Drawing for the job (mm, zero at the part's lowest x, y, z). A direction names the side the tool comes from. Round coordinates to 2 decimals unless told otherwise and drop trailing zeros. Write each loop counter-clockwise with the first axis right and the second up, starting at its lowest first coordinate (ties: lowest second). Pieces come first, ordered by that corner, then holes. Notation, with made-up numbers: (44, 66) - (52, 66) arc R31 cw to (52, 102) - close; hole circle Ø11 at (31.25, 47.5). An arc over 180 degrees is marked (long way). One line per question, with ' | ' between items.
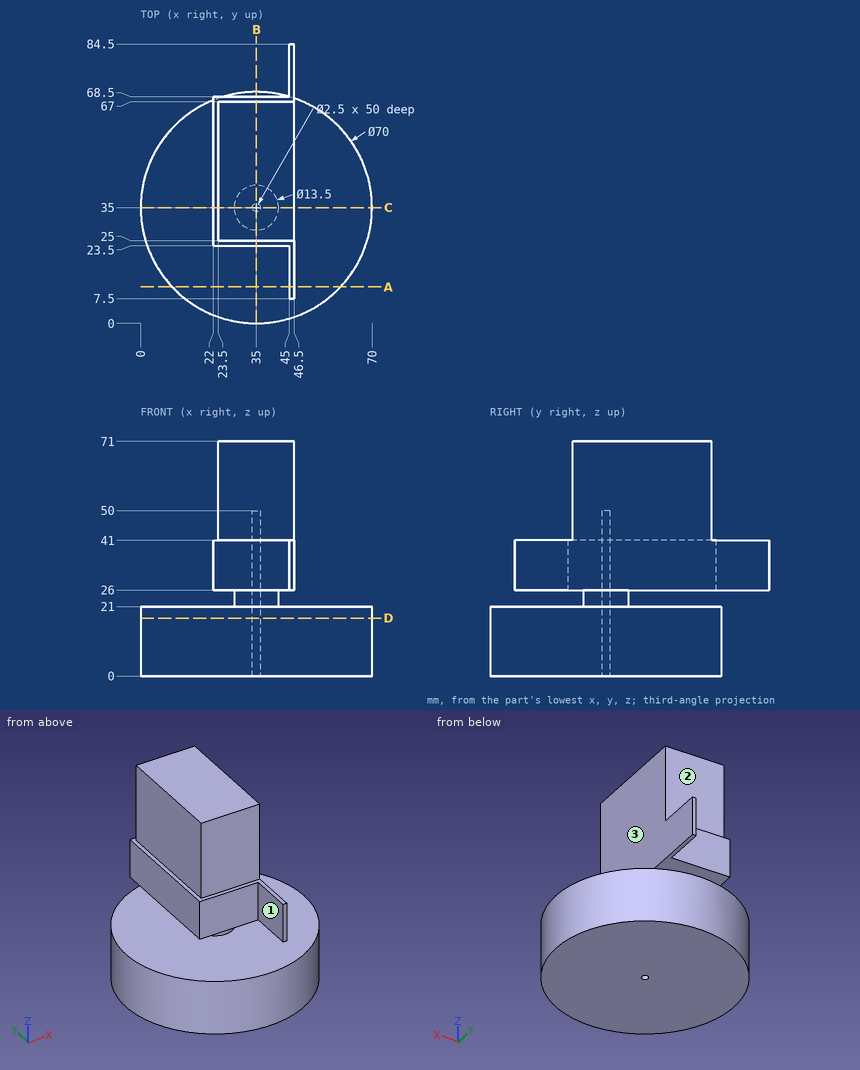
Q1. Drill centre lines: L1, parallel to Z at x = 43.5, y = 35.5; L2, parallel to Y at x = 35, z = 19; L3, parallel to Y at x = 35, z = 38. Where is each one in solid material? Low to high. Write a range as from..to.
Found:
L1: 0..21, 26..71 | L2: 0..33.75, 36.25..70 | L3: 23.5..33.75, 36.25..68.5
Q2. Which spindle directions (+Z, -Z, +X, -X, +Y, -Y) get a long thin tool onto all of the face, cutting with end or side? Do the marked faces 1, 2 and 3. Say none if no direction does.
Found:
face 1: +Z, -X, -Y | face 2: +Z, +X, -X, +Y | face 3: +Z, +X, +Y, -Y
Q3. Saw through at C-C, the plane y = 35. List the corners of the cut face in (x, z).
Found:
outline: (0, 0) - (33.75, 0) - (33.75, 50) - (36.25, 50) - (36.25, 0) - (70, 0) - (70, 21) - (41.75, 21) - (41.75, 26) - (46.5, 26) - (46.5, 71) - (23.5, 71) - (23.5, 41) - (22, 41) - (22, 26) - (28.25, 26) - (28.25, 21) - (0, 21) - close
Q4. Drop flat-ended pins along their axis: pin 1 (2 mm diameter, centred on x = 15, z = 13.5, fed in from +Y); pin 2 (12 mm diameter, centred on y = 77, z = 35, fed in from -X); pin 3 (11.5 mm diameter, centred on x = 38.5, z = 63, fed in from +Y). Give the stop position or say it passes through.
Found:
pin 1: y = 64.39 | pin 2: x = 45 | pin 3: y = 67
Q5. Saw through at A-A, the plane y = 11. List the corners of the cut face in (x, z), then the cut area to 3 significant figures.
Found:
outline: (9.52, 0) - (60.48, 0) - (60.48, 21) - (9.52, 21) - close; (45, 26) - (46.5, 26) - (46.5, 41) - (45, 41) - close | area: 1,090 mm^2
Q6. Saw through at B-B, the plane x = 35. List the corners of the cut face in (y, z), then the cut area to 3 significant figures.
Found:
outline: (0, 0) - (33.75, 0) - (33.75, 50) - (36.25, 50) - (36.25, 0) - (70, 0) - (70, 21) - (41.75, 21) - (41.75, 26) - (68.5, 26) - (68.5, 41) - (67, 41) - (67, 71) - (25, 71) - (25, 41) - (23.5, 41) - (23.5, 26) - (28.25, 26) - (28.25, 21) - (0, 21) - close | area: 3,350 mm^2
Q7. Saw through at D-D, the plane z = 17.5. List the corners of the cut face in (x, y).
Found:
outline: circle Ø70 at (35, 35); hole circle Ø2.5 at (35, 35)
